Geometry check sheet. Reference: the model listing, model coordinates, mm. A direction names the side the tool comes from. Round coordinates to 2 decimals unless told otherwise and drop trailing zeros. Write each loop counter-clockwise with the first axis right and the second up, starting at its lowest first coordinate (ties: lowest second). Pieces come first, ordered by that corner, then holes. Notation, with made-up numbers: M 60.25,79 L 119.25,79 A16 cw 119.25,92 Z; hole C 24.5,-6.5 d1. An arc over 180 degrees is marked long. Use a Markdown table: item, result.
```python
from build123d import *

# Parameters (mm, degrees)
SKETCH1_R           = 12
BOSS_EXTRUDE1_DEPTH = 3
SKETCH2_R           = 5
BOSS_EXTRUDE2_DEPTH = 15
CUT_EXTRUDE1_DEPTH  = 15
SKETCH4_R           = 1.5
CUT_EXTRUDE2_DEPTH  = 5


with BuildPart() as part:
    # Sketch1 → Boss-Extrude1 (new body)
    with BuildSketch(Plane.XY):
        Circle(SKETCH1_R)
    extrude(amount=BOSS_EXTRUDE1_DEPTH)

    # Sketch2 → Boss-Extrude2 (add)
    with BuildSketch(Plane.XY):
        Circle(SKETCH2_R)
    extrude(amount=BOSS_EXTRUDE2_DEPTH)

    # Sketch3 → Cut-Extrude1 (cut)
    with BuildSketch(Plane.XY):
        with BuildLine():
            Line((-0.065110368, 2.2008), (1.421576364, 2.2008))
            ThreePointArc((1.421576364, 2.2008), (0, -2.62), (-1.421576364, 2.2008))
            Line((-1.421576364, 2.2008), (-0.065110368, 2.2008))
        make_face()
    extrude(amount=CUT_EXTRUDE1_DEPTH, mode=Mode.SUBTRACT)

    # Sketch4 → Cut-Extrude2 (cut)
    with BuildSketch(Plane.XY):
        with Locations((-9, 0)):
            Circle(SKETCH4_R)
        with Locations((0, 9)):
            Circle(SKETCH4_R)
        with Locations((9, 0)):
            Circle(SKETCH4_R)
        with Locations((0, -9)):
            Circle(SKETCH4_R)
    extrude(amount=CUT_EXTRUDE2_DEPTH, mode=Mode.SUBTRACT)


solid = part.part
```
Item 1: Go/stop test with flat-tipped pins: pin 1 (12 mm diameter, centred on x = -9, y = -8.5, fed in from +Z); pin 2 (5 mm diameter, centred on x = -3, z = 5, fed in from -Y); pin 3 (6 mm diameter, centred on x = 0, z = 12, fed in from +Y). Record where each tip stops, or that it passes through.
Outcome:
| item | result |
|---|---|
| pin 1 | stops at z = 3 |
| pin 2 | stops at y = -11.91 |
| pin 3 | stops at y = 5 |
Item 2: Material ranges on line 1 along Z through (x, y) = (7.75, -5.5); line 2 along Y through (x, z) = (2.25, 14.5); line 3 along Y through (x, z) = (-0.25, 11), recorded low to high. Write a range as from..to.
Outcome:
| item | result |
|---|---|
| line 1 | z = 0..3 |
| line 2 | y = -4.47..-1.34, 1.34..4.47 |
| line 3 | y = -4.99..-2.61, 2.2..4.99 |
Item 3: Mould release check, pull along X, two halves, no side actions. Record for faces 3 (the face through (-0.325, 7.536, 1.479)), 4 (the face through (5.2, 0.2, 3)), 5 (the face through (-1.08, -4.88, 8.92)): +X half, -X half, draft (parallel to the pull), parting line (faces both ways), or undercut.
Outcome:
| item | result |
|---|---|
| face 3 | undercut |
| face 4 | draft |
| face 5 | parting line |
Item 4: Cross-section at B-B, the plane x = 0. Record the cut outline in (y, z), and give its area (3 significant figures).
Outcome:
| item | result |
|---|---|
| outline | M -12,0 L -10.5,0 L -10.5,3 L -12,3 Z; M -7.5,0 L -2.62,0 L -2.62,15 L -5,15 L -5,3 L -7.5,3 Z; M 2.2,0 L 7.5,0 L 7.5,3 L 5,3 L 5,15 L 2.2,15 Z; M 10.5,0 L 12,0 L 12,3 L 10.5,3 Z |
| area | 102 mm2 |
Item 5: Cross-section at C-C, the plane x = -9. Record the cut outline in (y, z).
Outcome:
| item | result |
|---|---|
| outline | M -7.94,0 L -1.5,0 L -1.5,3 L -7.94,3 Z; M 1.5,0 L 7.94,0 L 7.94,3 L 1.5,3 Z |
Item 6: Cross-section at A-A, the plane y = 0. Record the cut outline in (x, z).
Outcome:
| item | result |
|---|---|
| outline | M -12,0 L -10.5,0 L -10.5,3 L -12,3 Z; M -7.5,0 L -2.62,0 L -2.62,15 L -5,15 L -5,3 L -7.5,3 Z; M 2.62,0 L 7.5,0 L 7.5,3 L 5,3 L 5,15 L 2.62,15 Z; M 10.5,0 L 12,0 L 12,3 L 10.5,3 Z |
Item 7: Access from +Z, -Z, +X, -X, +Y, -Y to the whole of each face (thin tool, end or side, straight path). Record for faces 1 (the face through (2, -2, 15)), 2 (the face through (0, 2.201, 7)).
Outcome:
| item | result |
|---|---|
| face 1 | +Z, +X, -X, +Y, -Y |
| face 2 | +Z, -Z |
